Geometry: final body of the model. Coordinates: model frame, mm. A direction names the side the tool comes from. Round coordinates to 2 decimals unless told otherwise and drop trailing zeros. Loops run counter-clockwise (first coordinate to the right, second up) from the corner with the lowest first, then second, coordinate; pieces in that order, holes last. Notation, with made-up numbers: (-7.5, 37.25) -> (11.5, 37.25) arc R15 ccw to (11.5, 59.25) -> close; hole circle Ø8 at (80.5, 23.25). An arc over 180 degrees is marked (long way). Answer in a Markdown table with one row per item.
```python
from build123d import *

# Parameters (mm, degrees)
F0_R     = 2.1463
F1_DEPTH = 10


with BuildPart() as f1:
    # F0 (on Front) → F1 (new body)
    with BuildSketch(Plane.XZ):
        with BuildLine():
            Line((-9.75241, 4.759444), (-12.019248, 4.759444))
            ThreePointArc((-12.019248, 4.759444), (-13.166227, 4.987592), (-14.138589, 5.637303))
            Line((-14.138589, 5.637303), (-16.393426, 7.892141))
            ThreePointArc((-16.393426, 7.892141), (-16.575125, 8.805603), (-15.800729, 9.323038))
            Line((-15.800729, 9.323038), (-13.692529, 9.323038))
            ThreePointArc((-13.692529, 9.323038), (-13.477003, 9.412312), (-13.387729, 9.627838))
            Line((-13.387729, 9.627838), (-13.387729, 10.339038))
            ThreePointArc((-13.387729, 10.339038), (-13.618353, 10.895814), (-14.175129, 11.126438))
            Line((-14.175129, 11.126438), (-18.874129, 11.126438))
            ThreePointArc((-18.874129, 11.126438), (-20.29301, 10.538718), (-20.880729, 9.119838))
            Line((-20.880729, 9.119838), (-20.880729, 4.420838))
            ThreePointArc((-20.880729, 4.420838), (-20.650105, 3.864062), (-20.093329, 3.633438))
            Line((-20.093329, 3.633438), (-19.382129, 3.633438))
            ThreePointArc((-19.382129, 3.633438), (-19.166603, 3.722712), (-19.077329, 3.938238))
            Line((-19.077329, 3.938238), (-19.077329, 6.046438))
            ThreePointArc((-19.077329, 6.046438), (-18.559895, 6.820834), (-17.646432, 6.639135))
            Line((-17.646432, 6.639135), (-15.391595, 4.384297))
            ThreePointArc((-15.391595, 4.384297), (-14.741884, 3.411936), (-14.513736, 2.264957))
            Line((-14.513736, 2.264957), (-14.513736, -0.001881))
            ThreePointArc((-14.513736, -0.001881), (-14.741884, -1.14886), (-15.391595, -2.121222))
            Line((-15.391595, -2.121222), (-17.646432, -4.376059))
            ThreePointArc((-17.646432, -4.376059), (-18.559895, -4.557758), (-19.077329, -3.783362))
            Line((-19.077329, -3.783362), (-19.077329, -1.675162))
            ThreePointArc((-19.077329, -1.675162), (-19.166603, -1.459636), (-19.382129, -1.370362))
            Line((-19.382129, -1.370362), (-20.093329, -1.370362))
            ThreePointArc((-20.093329, -1.370362), (-20.650105, -1.600986), (-20.880729, -2.157762))
            Line((-20.880729, -2.157762), (-20.880729, -6.856762))
            ThreePointArc((-20.880729, -6.856762), (-20.29301, -8.275643), (-18.874129, -8.863362))
            Line((-18.874129, -8.863362), (-14.175129, -8.863362))
            ThreePointArc((-14.175129, -8.863362), (-13.618353, -8.632738), (-13.387729, -8.075962))
            Line((-13.387729, -8.075962), (-13.387729, -7.364762))
            ThreePointArc((-13.387729, -7.364762), (-13.477003, -7.149236), (-13.692529, -7.059962))
            Line((-13.692529, -7.059962), (-15.800729, -7.059962))
            ThreePointArc((-15.800729, -7.059962), (-16.575125, -6.542528), (-16.393426, -5.629065))
            Line((-16.393426, -5.629065), (-14.138589, -3.374228))
            ThreePointArc((-14.138589, -3.374228), (-13.166227, -2.724517), (-12.019248, -2.496368))
            Line((-12.019248, -2.496368), (-9.75241, -2.496368))
            ThreePointArc((-9.75241, -2.496368), (-8.605431, -2.724517), (-7.63307, -3.374228))
            Line((-7.63307, -3.374228), (-5.378232, -5.629065))
            ThreePointArc((-5.378232, -5.629065), (-5.196534, -6.542528), (-5.970929, -7.059962))
            Line((-5.970929, -7.059962), (-8.079129, -7.059962))
            ThreePointArc((-8.079129, -7.059962), (-8.294656, -7.149236), (-8.383929, -7.364762))
            Line((-8.383929, -7.364762), (-8.383929, -8.075962))
            ThreePointArc((-8.383929, -8.075962), (-8.153305, -8.632738), (-7.596529, -8.863362))
            Line((-7.596529, -8.863362), (5.814671, -8.863362))
            ThreePointArc((5.814671, -8.863362), (6.371447, -8.632738), (6.602071, -8.075962))
            Line((6.602071, -8.075962), (6.602071, -7.364762))
            ThreePointArc((6.602071, -7.364762), (6.512797, -7.149236), (6.297271, -7.059962))
            Line((6.297271, -7.059962), (4.189071, -7.059962))
            ThreePointArc((4.189071, -7.059962), (3.414675, -6.542528), (3.596374, -5.629065))
            Line((3.596374, -5.629065), (5.851211, -3.374228))
            ThreePointArc((5.851211, -3.374228), (6.823573, -2.724517), (7.970552, -2.496368))
            Line((7.970552, -2.496368), (10.23739, -2.496368))
            ThreePointArc((10.23739, -2.496368), (11.384369, -2.724517), (12.35673, -3.374228))
            Line((12.35673, -3.374228), (14.611568, -5.629065))
            ThreePointArc((14.611568, -5.629065), (14.793266, -6.542528), (14.018871, -7.059962))
            Line((14.018871, -7.059962), (11.910671, -7.059962))
            ThreePointArc((11.910671, -7.059962), (11.695144, -7.149236), (11.605871, -7.364762))
            Line((11.605871, -7.364762), (11.605871, -8.075962))
            ThreePointArc((11.605871, -8.075962), (11.836495, -8.632738), (12.393271, -8.863362))
            Line((12.393271, -8.863362), (17.092271, -8.863362))
            ThreePointArc((17.092271, -8.863362), (18.511151, -8.275643), (19.098871, -6.856762))
            Line((19.098871, -6.856762), (19.098871, -2.157762))
            ThreePointArc((19.098871, -2.157762), (18.868247, -1.600986), (18.311471, -1.370362))
            Line((18.311471, -1.370362), (17.600271, -1.370362))
            ThreePointArc((17.600271, -1.370362), (17.384744, -1.459636), (17.295471, -1.675162))
            Line((17.295471, -1.675162), (17.295471, -3.783362))
            ThreePointArc((17.295471, -3.783362), (16.778036, -4.557758), (15.864574, -4.376059))
            Line((15.864574, -4.376059), (13.609736, -2.121222))
            ThreePointArc((13.609736, -2.121222), (12.960025, -1.14886), (12.731877, -0.001881))
            Line((12.731877, -0.001881), (12.731877, 2.264957))
            ThreePointArc((12.731877, 2.264957), (12.960025, 3.411936), (13.609736, 4.384297))
            Line((13.609736, 4.384297), (15.864574, 6.639135))
            ThreePointArc((15.864574, 6.639135), (16.778036, 6.820834), (17.295471, 6.046438))
            Line((17.295471, 6.046438), (17.295471, 3.938238))
            ThreePointArc((17.295471, 3.938238), (17.384744, 3.722712), (17.600271, 3.633438))
            Line((17.600271, 3.633438), (18.311471, 3.633438))
            ThreePointArc((18.311471, 3.633438), (18.868247, 3.864062), (19.098871, 4.420838))
            Line((19.098871, 4.420838), (19.098871, 9.119838))
            ThreePointArc((19.098871, 9.119838), (18.511151, 10.538718), (17.092271, 11.126438))
            Line((17.092271, 11.126438), (12.393271, 11.126438))
            ThreePointArc((12.393271, 11.126438), (11.836495, 10.895814), (11.605871, 10.339038))
            Line((11.605871, 10.339038), (11.605871, 9.627838))
            ThreePointArc((11.605871, 9.627838), (11.695144, 9.412312), (11.910671, 9.323038))
            Line((11.910671, 9.323038), (14.018871, 9.323038))
            ThreePointArc((14.018871, 9.323038), (14.793266, 8.805603), (14.611568, 7.892141))
            Line((14.611568, 7.892141), (12.35673, 5.637303))
            ThreePointArc((12.35673, 5.637303), (11.384369, 4.987592), (10.23739, 4.759444))
            Line((10.23739, 4.759444), (7.970552, 4.759444))
            ThreePointArc((7.970552, 4.759444), (6.823573, 4.987592), (5.851211, 5.637303))
            Line((5.851211, 5.637303), (3.596374, 7.892141))
            ThreePointArc((3.596374, 7.892141), (3.414675, 8.805603), (4.189071, 9.323038))
            Line((4.189071, 9.323038), (6.297271, 9.323038))
            ThreePointArc((6.297271, 9.323038), (6.512797, 9.412312), (6.602071, 9.627838))
            Line((6.602071, 9.627838), (6.602071, 10.339038))
            ThreePointArc((6.602071, 10.339038), (6.371447, 10.895814), (5.814671, 11.126438))
            Line((5.814671, 11.126438), (-7.596529, 11.126438))
            ThreePointArc((-7.596529, 11.126438), (-8.153305, 10.895814), (-8.383929, 10.339038))
            Line((-8.383929, 10.339038), (-8.383929, 9.627838))
            ThreePointArc((-8.383929, 9.627838), (-8.294656, 9.412312), (-8.079129, 9.323038))
            Line((-8.079129, 9.323038), (-5.970929, 9.323038))
            ThreePointArc((-5.970929, 9.323038), (-5.196534, 8.805603), (-5.378232, 7.892141))
            Line((-5.378232, 7.892141), (-7.63307, 5.637303))
            ThreePointArc((-7.63307, 5.637303), (-8.605431, 4.987592), (-9.75241, 4.759444))
        make_face()
        with Locations((-10.885829, 1.131538)):
            Circle(F0_R, mode=Mode.SUBTRACT)
        with BuildLine():
            Line((-7.257923, -0.001881), (-7.257923, 2.264957))
            ThreePointArc((-7.257923, 2.264957), (-7.029775, 3.411936), (-6.380064, 4.384297))
            Line((-6.380064, 4.384297), (-1.83051, 8.933851))
            ThreePointArc((-1.83051, 8.933851), (-0.890929, 9.323038), (0.048652, 8.933851))
            Line((0.048652, 8.933851), (4.598205, 4.384297))
            ThreePointArc((4.598205, 4.384297), (5.247916, 3.411936), (5.476064, 2.264957))
            Line((5.476064, 2.264957), (5.476064, -0.001881))
            ThreePointArc((5.476064, -0.001881), (5.247916, -1.14886), (4.598205, -2.121222))
            Line((4.598205, -2.121222), (0.048652, -6.670775))
            ThreePointArc((0.048652, -6.670775), (-0.890929, -7.059962), (-1.83051, -6.670775))
            Line((-1.83051, -6.670775), (-6.380064, -2.121222))
            ThreePointArc((-6.380064, -2.121222), (-7.029775, -1.14886), (-7.257923, -0.001881))
        make_face(mode=Mode.SUBTRACT)
        with Locations((9.103971, 1.131538)):
            Circle(F0_R, mode=Mode.SUBTRACT)
    extrude(amount=F1_DEPTH)


solid = f1.part
```
Item 1: First-contact query: P1, Ø4, axis at x = -10, z = 8.5, coming from the -Y side; P2, Ø0.7, axis at y = -5, z = 0.5, coming from the +X side; P3, Ø0.7, axis at x = 9, y = -7, coming from the -Z side; P4, Ø1.1, axis at y = -7, z = 0.5, coming from the -X side. Flat tips, straight axial feed; report the tip coordinate or a pass-through.
Ans:
| item | result |
|---|---|
| P1 | y = -10 |
| P2 | x = 12.73 |
| P3 | z = -2.5 |
| P4 | x = -14.51 |
Item 2: Section query D-D, the plane z = -0.5. Output: boundary loops of the cut face in (x, y).
Ans:
| item | result |
|---|---|
| outline | (-14.56, -10) -> (-12.28, -10) -> (-12.28, 0) -> (-14.56, 0) -> close; (-9.49, -10) -> (-7.22, -10) -> (-7.22, 0) -> (-9.49, 0) -> close; (5.43, -10) -> (7.71, -10) -> (7.71, 0) -> (5.43, 0) -> close; (10.5, -10) -> (12.77, -10) -> (12.77, 0) -> (10.5, 0) -> close |
Item 3: Mould query, pull axis X, two halves, no side actions, for faces 1 (the flat face through (-1, -5, 11.126)), 2 (the flat face through (12.732, -5, 1)), 3 (the flat face through (-4.137, -4.93, 6.627)). Classes: released by +X, released by -X, zero draft, split by the parting line, or undercut.
Ans:
| item | result |
|---|---|
| face 1 | zero draft |
| face 2 | released by +X |
| face 3 | undercut |
Item 4: Section query B-B, the plane x = -1. Output: boundary loops of the cut face in (y, z), and give its area (3 significant figures).
Ans:
| item | result |
|---|---|
| outline | (-10, -8.86) -> (0, -8.86) -> (0, -7.06) -> (-10, -7.06) -> close; (-10, 9.32) -> (0, 9.32) -> (0, 11.13) -> (-10, 11.13) -> close |
| area | 36.2 mm2 |
Item 5: Section query A-A, the plane z = 1.5. Output: boundary loops of the cut face in (x, y), and give its area (3 significant figures).
Ans:
| item | result |
|---|---|
| outline | (-14.51, -10) -> (-13, -10) -> (-13, 0) -> (-14.51, 0) -> close; (-8.77, -10) -> (-7.26, -10) -> (-7.26, 0) -> (-8.77, 0) -> close; (5.48, -10) -> (6.99, -10) -> (6.99, 0) -> (5.48, 0) -> close; (11.22, -10) -> (12.73, -10) -> (12.73, 0) -> (11.22, 0) -> close |
| area | 60.5 mm2 |
Item 6: Set-up query: faces 4 (the flat face through (-6, -10, -3)), 5 (the flat face through (14.721, -4.93, 5.496)), 6 (the flat face through (-11, -5, 4.759)). Return all of +Z, -Z, +X, -X, +Y, -Y with unobstructed straight access to the full face (end or side cutting, diameter ignored); none if empty.
Ans:
| item | result |
|---|---|
| face 4 | +Z, -Z, +X, -X, -Y |
| face 5 | +Y, -Y |
| face 6 | +Z, +Y, -Y |
Item 7: Ray query, L1, parallel to X at y = -7.25, z = 6.75; L2, parallel to X at y = -0.75, z = -0.25; L3, parallel to Z at x = -13.5, y = -7. Return the intervals inside material, ascending.
Ans:
| item | result |
|---|---|
| L1 | -20.88 to -18.69, -17.78 to -15.25, -6.52 to -4.01, 2.23 to 4.74, 13.47 to 16, 16.91 to 19.1 |
| L2 | -14.52 to -12.53, -9.24 to -7.25, 5.47 to 7.46, 10.75 to 12.74 |
| L3 | -8.48 to -7.13, -2.89 to 5.15, 9.39 to 10.74 |
Item 8: Section query C-C, the plane y = -3.5. State how many separate pieces and enclosed holes the cut face has, and give its area (4 significant figures).
Ans:
| item | result |
|---|---|
| separate pieces | 1 |
| enclosed holes | 3 |
| area | 328.5 mm2 |
